Read the model definition and answer for the solid it produces. Units are mm, in the model's axes. A direction names the side the tool comes from. Round coordinates to 2 decimals unless told otherwise and drop trailing zeros. Order: outer loops, then holes, each group sorted by start corner. A loop starts at its lowest first (then second) coordinate and runs counter-clockwise, first axis right, second up. Notation, with made-up numbers: (35.5, -6) -> (74.5, -6) arc R23 cw to (74.5, 27) -> close; hole circle Ø4 at (9, 36.25). An arc over 180 degrees is marked (long way). Answer as a JSON object with one key per item and string values. Group by question number.
Item 1: For faces 1 (the flat face through (-3, -48.57, 3)), 2 (the flat face through (0, 1, 0)), determine the directions among +Z, -Z, +X, -X, +Y, -Y from which every point of the face is accessible in a straight line to the end or side of a thin tool.
Item 2: Section B-B, the plane y = 46.04 is taken. Write down the section's boundary in (x, z), plus the area to 3 significant figures.
Item 3: Given P1, Ø5, axis at x = 11.43, y = 46.04, coming from the -Z side; P2, Ø2.5, axis at x = 11.43, y = -46.04, coming from the +Z side; P3, Ø1.5, axis at x = -8.5, z = 4.5, coming from the -Y side, each flat-ended and moving along its own axis, determine where each tip first touches the part or whether it passes through.
Item 4: Section A-A, the plane z = 6.25 is taken. Write down the section's boundary in (x, y), plus the area to 3 significant figures.
Item 5: Consider probe 1 along Y at (x, z) = (-11.43, 7.5); probe 2 along Y at (x, z) = (-12, 5); probe 3 along X at (y, z) = (-71.5, 6). Determine where each line is inside the solid, lowest interval first. Write a range as from..to.
Item 6: The mould has two halves that part along X. Classify faces 3 (the flat face through (0, 1, 12.5)), 4 (the flat face through (-13.97, -1, 6)), 5 (the cylindrical face through (-12.12, -47.37, 6.16)): pulls with the +X half, pulls with the -X half, needs draft (parallel to the pull), parting line crosses it, or undercut.
Item 7: Section C-C, the plane x = 11.43 is taken. Write down the section's boundary in (y, z), plus the area to 3 significant figures.
Item 8: Section D-D, the plane x = 0 is taken. Write down the section's boundary in (y, z), plus the area to 3 significant figures.
from build123d import *

# Parameters (mm, degrees)
SKETCH1_W           = 27.94
SKETCH1_H           = 97.14
BOSS_EXTRUDE1_DEPTH = 12.5
SKETCH2_R           = 1.5
CUT_EXTRUDE1_DEPTH  = 23
SKETCH3_R           = 3.5
BOSS_EXTRUDE2_DEPTH = 45


with BuildPart() as part:
    # Sketch1 → Boss-Extrude1 (new body)
    with BuildSketch(Plane.XY):
        Rectangle(SKETCH1_W, SKETCH1_H)
    extrude(amount=BOSS_EXTRUDE1_DEPTH)

    # Sketch2 → Cut-Extrude1 (cut)
    with BuildSketch(Plane(origin=(0, 0, 0), x_dir=(-1, 0, 0), z_dir=(0, 0, -1))):
        with Locations((-11.43, 46.04)):
            Circle(SKETCH2_R)
        with Locations((-11.43, -46.04)):
            Circle(SKETCH2_R)
        with Locations((11.43, 46.04)):
            Circle(SKETCH2_R)
        with Locations((11.43, -46.04)):
            Circle(SKETCH2_R)
    extrude(amount=-CUT_EXTRUDE1_DEPTH, mode=Mode.SUBTRACT)

    # Sketch3 → Boss-Extrude2 (add)
    with BuildSketch(Plane.XZ.offset(48.57)):
        with Locations(Location((0, 6.25, 0), (0, 0, 90))):
            Circle(SKETCH3_R)
    extrude(amount=BOSS_EXTRUDE2_DEPTH)


solid = part.part
Values found:
{
 "1": {"face 1": "-Y", "face 2": "-Z, +X, -X, +Y, -Y"},
 "2": {"outline": "(-13.97, 0) -> (-12.93, 0) -> (-12.93, 12.5) -> (-13.97, 12.5) -> close; (-9.93, 0) -> (9.93, 0) -> (9.93, 12.5) -> (-9.93, 12.5) -> close; (12.93, 0) -> (13.97, 0) -> (13.97, 12.5) -> (12.93, 12.5) -> close", "area": "274 mm2"},
 "3": {"P1": "z = 0", "P2": "through", "P3": "y = -48.57"},
 "4": {"outline": "(-13.97, -48.57) -> (-3.5, -48.57) -> (-3.5, -93.57) -> (3.5, -93.57) -> (3.5, -48.57) -> (13.97, -48.57) -> (13.97, 48.57) -> (-13.97, 48.57) -> close; hole circle Ø3 at (-11.43, -46.04); hole circle Ø3 at (-11.43, 46.04); hole circle Ø3 at (11.43, -46.04); hole circle Ø3 at (11.43, 46.04)", "area": "3,000 mm2"},
 "5": {"probe 1": "-48.57..-47.54, -44.54..44.54, 47.54..48.57", "probe 2": "-48.57..-47.43, -44.65..44.65, 47.43..48.57", "probe 3": "-3.49..3.49"},
 "6": {"face 3": "needs draft", "face 4": "pulls with the -X half", "face 5": "undercut"},
 "7": {"outline": "(-48.57, 0) -> (-47.54, 0) -> (-47.54, 12.5) -> (-48.57, 12.5) -> close; (-44.54, 0) -> (44.54, 0) -> (44.54, 12.5) -> (-44.54, 12.5) -> close; (47.54, 0) -> (48.57, 0) -> (48.57, 12.5) -> (47.54, 12.5) -> close", "area": "1,140 mm2"},
 "8": {"outline": "(-93.57, 2.75) -> (-48.57, 2.75) -> (-48.57, 0) -> (48.57, 0) -> (48.57, 12.5) -> (-48.57, 12.5) -> (-48.57, 9.75) -> (-93.57, 9.75) -> close", "area": "1,530 mm2"}
}
